Could you check a few things on this model? Use its own coordinates, in mm. Face numbers are marked on the shaded views. A direction names the side the tool comes from. Coordinates: 2 decimals unless noted, no trailing zeros. Order: outer loops, then holes, each group sorted by start corner. A loop starts at its lowest first (then second) coordinate and runs counter-clockwise, first axis right, second up. Notation, with made-up numbers: (48, 70) - (105, 70) arc R25 ccw to (105, 87) - close; hole circle Ø1 at (49.5, 48.25). An arc over 180 degrees is marked (long way). One line per item, written item: value.
Autodesk Inventor part; units mm, degrees
ref_plane "YZ Plane" through (0, 0, 0) normal (1, 0, 0) x (0, 1, 0)
ref_plane "XZ Plane" through (0, 0, 0) normal (0, 1, 0) x (-1, 0, 0)
ref_plane "XY Plane" through (0, 0, 0) normal (0, 0, 1) x (1, 0, 0)
sketch "Sketch1" plane through (0, 0, 0) normal (0, 0, 1) x (1, 0, 0)
  line L0 (75, -100) -> (-75, -100)
  line L1 (-75, 100) -> (75, 100)
  line L2 (75, -100) -> (-75, 100) construction
  line L3 (-75, -100) -> (75, 100) construction
  line L4 (-165, -35) -> (-165, 35)
  line L5 (165, 35) -> (165, -35)
  line L6 (165, -35) -> (-165, 35) construction
  line L7 (-165, -35) -> (165, 35) construction
  line L8 (-75, -100) -> (-75, -35)
  line L9 (-75, 35) -> (-75, 100)
  line L10 (-165, 35) -> (-75, 35)
  line L11 (75, 35) -> (165, 35)
  line L12 (75, 100) -> (75, 35)
  line L13 (75, -35) -> (75, -100)
  line L14 (165, -35) -> (75, -35)
  line L15 (-75, -35) -> (-165, -35)
  line L16 (-65, 90) -> (65, 90)
  line L17 (65, 90) -> (65, 25)
  line L18 (65, 25) -> (155, 25)
  line L19 (155, 25) -> (155, -25)
  line L20 (155, -25) -> (65, -25)
  line L21 (65, -25) -> (65, -90)
  line L22 (65, -90) -> (-65, -90)
  line L23 (-65, -90) -> (-65, -25)
  line L24 (-65, -25) -> (-155, -25)
  line L25 (-155, -25) -> (-155, 25)
  line L26 (-155, 25) -> (-65, 25)
  line L27 (-65, 25) -> (-65, 90)
  line L28 (-142, 25) -> (-142, -25)
  line L29 (142, 25) -> (142, -25)
  point P0 (0, 0)
  point P1 (0, 0)
  point P2 (0, 0)
  point P3 (0, 0)
  point P4 (0, 0)
  dimension "d0" = 70
  dimension "d1" = 330
  dimension "d2" = 150
  dimension "d3" = 200
  dimension "d10" = 10
  dimension "d11" = 23
  dimension "d12" = 23
extrude "Extrusion1" add sketch "Sketch1" along normal mid plane 85 contours L0 L8 L15 L4 L10 L9 L1 L12 L11 L5 L14 L13 | L16 L17 L18 L29 L20 L21 L22 L23 L24 L28 L26 L27 | L28 L24 L25 L26 | L18 L19 L20 L29
sketch "Sketch2" plane through (0, 0, 0) normal (0, 1, 0) x (-1, 0, 0)
  line L0 (-150, 42.5) -> (-165, 27.5)
  line L1 (-165, -42.5) -> (-165, 42.5)
  line L2 (-165, -27.5) -> (-150, -42.5)
  line L3 (-165, -42.5) -> (-75, -42.5)
  line L4 (75, 42.5) -> (165, 42.5)
  line L5 (150, 42.5) -> (165, 27.5)
  line L6 (165, -42.5) -> (165, 42.5)
  line L7 (-165, -42.5) -> (165, -42.5)
  line L8 (150, -42.5) -> (165, -27.5)
  line L9 (-165, 42.5) -> (165, 42.5)
  line L10 (165, 0) -> (-165, 0) construction
  line L11 (-165, 42.5) -> (-165, -42.5) construction
  line L12 (-75, 42.5) -> (75, 42.5) construction
  line L13 (0, 42.5) -> (0, -42.5) construction
  line L14 (75, -42.5) -> (-75, -42.5) construction
  point P0 (0, 0)
  dimension "d6" = 15
  dimension "d7" = 45
extrude "Extrusion2" cut sketch "Sketch2" along normal through all both and the other way through all contours L0 L1 L9 | L2 L3 L1 | L4 L6 L5 | L6 L7 L8
extrude "Extrusion3" cut sketch "Sketch1" along normal mid plane 65 contours L16 L17 L18 L29 L20 L21 L22 L23 L24 L28 L26 L27
equation "\"d10\" = wall_thickness"
equation "\"d13\" = body_thickness - 2 * wall_thickness"
equation "\"wall_thickness\" = 10"
equation "\"body_thickness\" = 85"
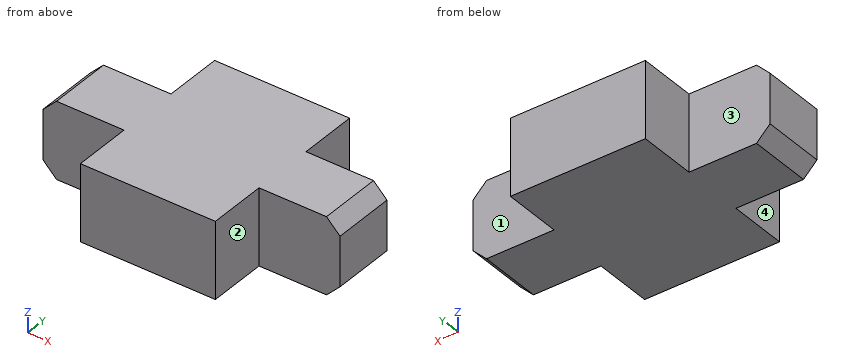
Item 1: I want a section at D-D on y = 2. Please give me the cut outline in (x, z), then the cut area to 3 significant figures.
Conclusion:
outline: (-165, -27.5) - (-150, -42.5) - (150, -42.5) - (165, -27.5) - (165, 27.5) - (150, 42.5) - (-150, 42.5) - (-165, 27.5) - close; hole (-142, -32.5) - (142, -32.5) - (142, 32.5) - (-142, 32.5) - close
area: 9,140 mm²
Item 2: If I drill on probe 1 along Y at (x, z) = (58.5, -9); probe 2 along X at (y, z) = (-31, 6.5); probe 3 along Z at (x, y) = (-40.5, -81), over which ranges is the centre line in solid material (lowest first)?
Conclusion:
probe 1: -100 to -90, 90 to 100
probe 2: -165 to -65, 65 to 165
probe 3: -42.5 to -32.5, 32.5 to 42.5
Item 3: I'm going to push flat-ended pins straight in: pin 1 Ø1.5 at (y, z) = (30.5, -30) entering from +X; pin 2 Ø8 at (y, z) = (63, 22) entering from -X; pin 3 Ø19.5 at (y, z) = (-75.5, -15) entering from +X. Where does each tip first touch, or does it pass through?
Conclusion:
pin 1: x = 163.25
pin 2: x = -75
pin 3: x = 75
Item 4: I want a section at A-A on y = 69. Please give me the cut outline in (x, z).
Conclusion:
outline: (-75, -42.5) - (75, -42.5) - (75, 42.5) - (-75, 42.5) - close; hole (-65, -32.5) - (65, -32.5) - (65, 32.5) - (-65, 32.5) - close
Item 5: I want a section at C-C on x = 14. Please give me the cut outline in (y, z), then the cut area to 3 significant figures.
Conclusion:
outline: (-100, -42.5) - (100, -42.5) - (100, 42.5) - (-100, 42.5) - close; hole (-90, -32.5) - (90, -32.5) - (90, 32.5) - (-90, 32.5) - close
area: 5,300 mm²
Item 6: For the marked faces 1, 2, 3 and 4, which set-ups out of +Z, -Z, +X, -X, +Y, -Y let a thin tool reach every point of the face, with its end or its side?
Conclusion:
face 1: +Z, -Z, +X, +Y
face 2: +Z, -Z, +X, -Y
face 3: +Z, -Z, -X, +Y
face 4: +Z, -Z, -X, -Y
Item 7: I want a section at B-B on z = 10.5. Please give me the cut outline in (x, y).
Conclusion:
outline: (-165, -35) - (-75, -35) - (-75, -100) - (75, -100) - (75, -35) - (165, -35) - (165, 35) - (75, 35) - (75, 100) - (-75, 100) - (-75, 35) - (-165, 35) - close; hole (-142, -25) - (-65, -25) - (-65, -90) - (65, -90) - (65, -25) - (142, -25) - (142, 25) - (65, 25) - (65, 90) - (-65, 90) - (-65, 25) - (-142, 25) - close
